Answer from the drawing. Dimensions are ordinates in mm from the lowest x, y and z of the part. Give positions to 0.01 mm unless a question says otherwise; leave off trailing zeros. Write each loop counter-clockwise with the first axis right and the second up, starting at its lowest first coordinate (ties: lowest second). Pieces come first, ordered by that corner, then holes.
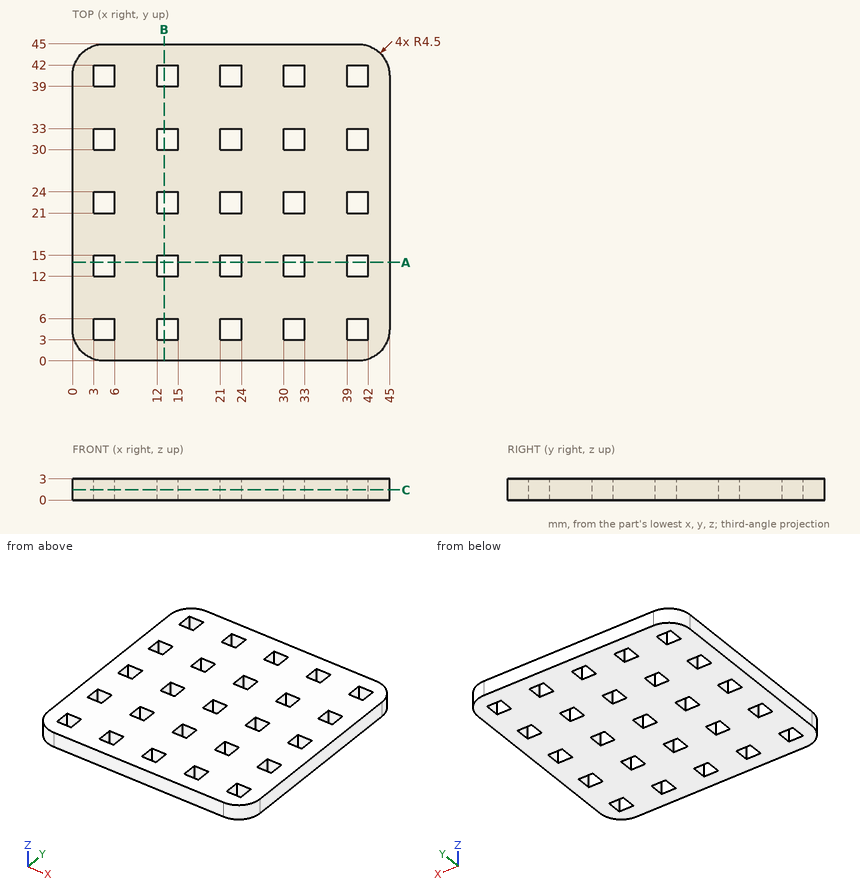
Item 1: Section C-C (z = 1.45) is taken. Give the number of separate pieces and of enclosed holes in the cut face, and give its area (3 significant figures).
Result set:
separate pieces: 1
enclosed holes: 25
area: 1,780 mm2
Item 2: Section A-A (y = 14) is taken. Write down the section's boundary in (x, z), and give its area (3 significant figures).
Result set:
outline: (0, 0) - (3, 0) - (3, 3) - (0, 3) - close; (6, 0) - (12, 0) - (12, 3) - (6, 3) - close; (15, 0) - (21, 0) - (21, 3) - (15, 3) - close; (24, 0) - (30, 0) - (30, 3) - (24, 3) - close; (33, 0) - (39, 0) - (39, 3) - (33, 3) - close; (42, 0) - (45, 0) - (45, 3) - (42, 3) - close
area: 90.0 mm2
Item 3: Find the intervals of material crossed by line 1 along Y through (x, z) = (31.5, 1.7); line 2 along Y through (x, z) = (43.5, 1), in increasing order.
Result set:
line 1: y = 0 to 3, 6 to 12, 15 to 21, 24 to 30, 33 to 39, 42 to 45
line 2: y = 1.15 to 43.85
